CAD build for the part. Positions are in the model's coordinates, mm. Round coordinates to 2 decimals unless told otherwise and drop trailing zeros. Loops run counter-clockwise (first coordinate to the right, second up) from the corner with the lowest first, then second, coordinate; pieces in that order, holes last.
```python
from build123d import *

# Parameters (mm, degrees)
SKETCH3_R           = 21.082
BOSS_EXTRUDE1_DEPTH = 6.35
CUT_EXTRUDE1_DEPTH  = 722.250266796
FILLET1_R           = 152.4
SKETCH5_R           = 21.971
CUT_EXTRUDE2_DEPTH  = 632.548321209


with BuildPart() as part:
    # Sketch3 → Boss-Extrude1 (new body)
    with BuildSketch(Plane(origin=(0, 0, 0), x_dir=(1, 0, 0), z_dir=(0, 1, 0))):
        Polygon((-534.293160191, 43.478424236), (-229.493160191, -484.450661911), (229.493160191, -484.450661911), (534.293160191, 43.478424236), (304.8, 440.972237675), (-304.8, 440.972237675), align=None)
        with Locations(Location((-352.63709, -203.595118838, 0), (0, 0, 270))):
            Circle(SKETCH3_R, mode=Mode.SUBTRACT)
        with Locations(Location((352.63709, -203.595118838, 0), (0, 0, 270))):
            Circle(SKETCH3_R, mode=Mode.SUBTRACT)
        with Locations(Location((0, 407.190237675, 0), (0, 0, 270))):
            Circle(SKETCH3_R, mode=Mode.SUBTRACT)
    extrude(amount=BOSS_EXTRUDE1_DEPTH)

    # Sketch4 → Cut-Extrude1 (cut, through all)
    with BuildSketch(Plane(origin=(0, 6.35, 0), x_dir=(1, 0, 0), z_dir=(0, 1, 0))):
        Polygon((-187.482425301, 440.972237675), (-475.634372841, -58.121575764), (-534.293160191, 43.478424236), (-304.8, 440.972237675), align=None)
        Polygon((304.8, 440.972237675), (534.293160191, 43.478424236), (475.634372841, -58.121575764), (187.482425301, 440.972237675), align=None)
        Polygon((229.493160191, -484.450661911), (-229.493160191, -484.450661911), (-288.15194754, -382.850661911), (288.15194754, -382.850661911), align=None)
    extrude(amount=-CUT_EXTRUDE1_DEPTH, mode=Mode.SUBTRACT)

    # Fillet1
    fillet1_edges = [part.edges().sort_by_distance(p)[0] for p in [
        (288.15194754, 3.175, 382.850661911),
        (-288.15194754, 3.175, 382.850661911),
        (187.482425301, 3.175, -440.972237675),
        (475.634372841, 3.175, 58.121575764),
        (-187.482425301, 3.175, -440.972237675),
        (-475.634372841, 3.175, 58.121575764),
    ]]
    fillet(fillet1_edges, radius=FILLET1_R)

    # Sketch5 → Cut-Extrude2 (cut, through all)
    with BuildSketch(Plane(origin=(0, 6.35, 0), x_dir=(1, 0, 0), z_dir=(0, 1, 0))):
        with Locations(Location((0, 407.190237675, 0), (0, 0, 270))):
            Circle(SKETCH5_R)
        with Locations(Location((352.63709, -203.595118838, 0), (0, 0, 270))):
            Circle(SKETCH5_R)
        with Locations(Location((-352.63709, -203.595118838, 0), (0, 0, 270))):
            Circle(SKETCH5_R)
    extrude(amount=-CUT_EXTRUDE2_DEPTH, mode=Mode.SUBTRACT)


solid = part.part
```
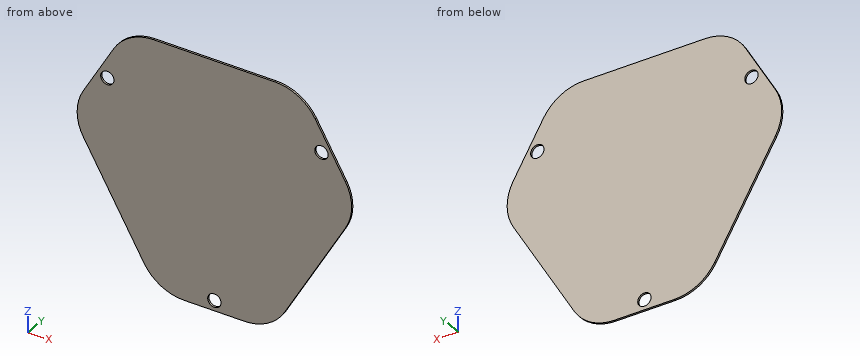
Item 1: Cut at B-B, the plane y = 2.25. Give the cut face in (x, z), plus the area to 3 significant figures.
Answers follow:
outline: (-431.64, -18.08) - (-231.48, -364.77) arc R152.4 ccw to (-99.49, -440.97) - (99.49, -440.97) arc R152.4 ccw to (231.48, -364.77) - (431.64, -18.08) arc R152.4 ccw to (431.64, 134.32) - (332.15, 306.65) arc R152.4 ccw to (200.16, 382.85) - (-200.16, 382.85) arc R152.4 ccw to (-332.15, 306.65) - (-431.64, 134.32) arc R152.4 ccw to start; hole circle Ø43.94 at (-352.64, 203.6); hole circle Ø43.94 at (0, -407.19); hole circle Ø43.94 at (352.64, 203.6)
area: 567,000 mm2
Item 2: Flat gauge pins, fed straight in: P1, Ø2, axis at x = -148, z = 235.5, coming from the -Y side; P2, Ø1, axis at x = -104.5, y = 3, coming from the -Z side. Where does each tip first touch, or does it go through?
Answers follow:
P1: stops at y = 0
P2: stops at z = -440.91
Item 3: Cut at C-C, the plane x = -257. Give the cut face in (y, z).
Answers follow:
outline: (0, -320.56) - (6.35, -320.56) - (6.35, 371.86) - (0, 371.86) - close
Item 4: Probe line 1 (X direction, y = 3.5, z = -272.5); line 2 (X direction, y = 2, z = -112); line 3 (Z direction, x = -217, y = 2.5). List the from-to ranges inside material, lowest first.
Answers follow:
line 1: x = -284.75 to 284.75
line 2: x = -377.41 to 377.41
line 3: z = -385.62 to 381.92
Item 5: Cut at D-D, the plane z = -136.5. Give the cut face in (x, y).
Answers follow:
outline: (-363.27, 0) - (363.27, 0) - (363.27, 6.35) - (-363.27, 6.35) - close
Item 6: Cut at A-A, the plane x = 0. Give the cut face in (y, z).
Answers follow:
outline: (0, -440.97) - (6.35, -440.97) - (6.35, -429.16) - (0, -429.16) - close; (0, -385.22) - (6.35, -385.22) - (6.35, 382.85) - (0, 382.85) - close
